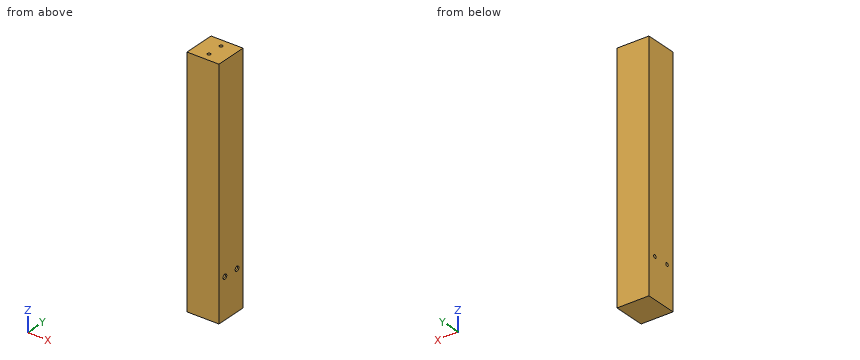
Solid Edge part; units mm, degrees
sketch "Sketch1" plane through (0, 0, 0) normal (0, 0, 1) x (1, 0, 0)
  line L0 (0, 0) -> (0, 40)
  line L1 (40, 40) -> (0, 40)
  line L2 (40, 0) -> (40, 40)
  line L3 (0, 0) -> (40, 0)
extrude "Protrusion1" add sketch "Sketch1" along normal blind 300
hole "Bohrung_1" at (20, 10, 300) direction (0, 0, -1) diameter 4.134 depth 40 tip angle 118
hole "Hole1" at (20, 30, 300) direction (0, 0, -1) diameter 4.134 depth 40 tip angle 118
hole "Bohrung_3" at (40, 10, 50) direction (-1, 0, 0) diameter 4.134 end through all start chamfer 1 start chamfer angle 45
hole "Hole2" at (40, 30, 50) direction (-1, 0, 0) diameter 4.134 end through all start chamfer 1 start chamfer angle 45
The model under review builds one solid part; all positions refer to its coordinate system, in mm. Coordinates: 2 decimals unless noted, no trailing zeros. Write each loop counter-clockwise with the first axis right and the second up, starting at its lowest first coordinate (ties: lowest second). Pieces come first, ordered by that corner, then holes. Notation, with made-up numbers: (17.25, 53) - (33.25, 53) arc R11 cw to (33.25, 65) - close; hole circle Ø10 at (-9, 73). An arc over 180 degrees is marked (long way). Answer in a Markdown table with one row per item. Add a question column.
Q1. Consider section A-A on z = 278. Give the boundary of the cut face in (x, y), then the cut area to 3 significant figures.
Q2. Clearance check with flat-ended pins moving along their axes: pin 1 (6 mm diameter, centred on x = 35.5, y = 20, fed in from -Z); pin 2 (3.5 mm diameter, centred on y = 10, z = 50, fed in from +X); pin 3 (5 mm diameter, centred on y = 30, z = 50, fed in from +X). State where each tip first meets the part, or that it passes through.
Q3. To check wall thickness, follow line 1 along Y through (x, z) = (31, 50); line 2 along Z through (x, y) = (8, 10); line 3 along Z through (x, y) = (20, 10). State the ranges of each line that lie inside material, in increasing order. Write a range as from..to.
Answers below:
| question | item | result |
|---|---|---|
| 1 | outline | (0, 0) - (40, 0) - (40, 40) - (0, 40) - close; hole circle Ø4.13 at (20, 10); hole circle Ø4.13 at (20, 30) |
| 1 | area | 1,570 mm² |
| 2 | pin 1 | z = 0 |
| 2 | pin 2 | through |
| 2 | pin 3 | x = 39.43 |
| 3 | line 1 | 0..7.93, 12.07..27.93, 32.07..40 |
| 3 | line 2 | 0..47.93, 52.07..300 |
| 3 | line 3 | 0..47.93, 52.07..258.76 |
